The figure shows three views and two pictorial views of one solid part (mm, origin at its lowest corner). Answer the questions. Coordinates: 2 decimals unless noted, no trailing zeros. Loops run counter-clockwise (first coordinate to the right, second up) from the corner with the lowest first, then second, coordinate; pieces in that order, holes last. Notation, with made-up numbers: (18, 12.25) -> (74, 12.25) arc R24 ccw to (74, 38.25) -> close; hole circle Ø7 at (6.25, 75.5). An arc over 180 degrees is marked (long way). Answer in a Markdown table with one row per item.
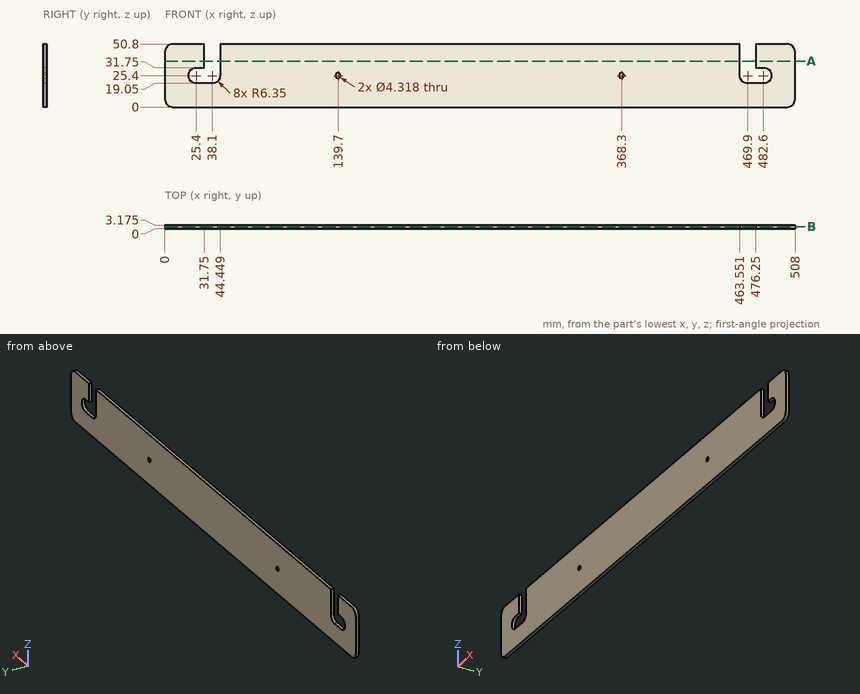
Item 1: A cutting plane is placed at B-B, the plane y = 1.9. Determine the outline of the cut face in (x, z).
Findings below:
| item | result |
|---|---|
| outline | (0, 6.35) arc R6.35 ccw to (6.35, 0) -> (501.65, 0) arc R6.35 ccw to (508, 6.35) -> (508, 44.45) arc R6.35 ccw to (501.65, 50.8) -> (476.25, 50.8) -> (476.25, 31.75) -> (482.6, 31.75) arc R6.35 cw to (482.6, 19.05) -> (469.9, 19.05) arc R6.35 cw to (463.55, 25.51) -> (463.55, 50.8) -> (44.45, 50.8) -> (44.45, 25.51) arc R6.35 cw to (38.1, 19.05) -> (25.4, 19.05) arc R6.35 cw to (25.4, 31.75) -> (31.75, 31.75) -> (31.75, 50.8) -> (6.35, 50.8) arc R6.35 ccw to (0, 44.45) -> close; hole circle Ø4.32 at (139.7, 25.4); hole circle Ø4.32 at (368.3, 25.4) |
Item 2: A cutting plane is placed at A-A, the plane z = 37. Determine the outline of the cut face in (x, y) (3 decimals), plus the area to 3 significant figures.
Findings below:
| item | result |
|---|---|
| outline | (0, 0) -> (31.75, 0) -> (31.75, 3.175) -> (0, 3.175) -> close; (44.449, 0) -> (463.551, 0) -> (463.551, 3.175) -> (44.449, 3.175) -> close; (476.25, 0) -> (508, 0) -> (508, 3.175) -> (476.25, 3.175) -> close |
| area | 1,530 mm2 |
Item 3: Find the intervals of material crossed by probe 1 along X at (y, z) = (2.55, 32.5); probe 2 along Z at (x, y) = (368.3, 1.65), in increasing order.
Findings below:
| item | result |
|---|---|
| probe 1 | x = 0 to 31.75, 44.45 to 463.55, 476.25 to 508 |
| probe 2 | z = 0 to 23.24, 27.56 to 50.8 |
Item 4: A flat-ended cylindrical pin translates along its axis: pin 1 Ø4 at (x, z) = (139.7, 25.4) entering from +Y. Find the tip coordinate at first contact, or state that the pin passes through.
Findings below:
| item | result |
|---|---|
| pin 1 | passes through |
